Verification items for the finished model (mm, model axes). A direction names the side the tool comes from. Round coordinates to 2 decimals unless told otherwise and drop trailing zeros. Write each loop counter-clockwise with the first axis right and the second up, starting at its lowest first coordinate (ties: lowest second). Pieces come first, ordered by that corner, then holes. Notation, with made-up numbers: (43.5, 74) -> (49.5, 74) arc R23 ccw to (49.5, 96) -> close; hole circle Ø4 at (50, -27). An arc over 180 degrees is marked (long way). Use CSV: the item, a comma, the result in double quotes.
Autodesk Inventor part; units mm, degrees
ref_plane "YZ Plane" through (0, 0, 0) normal (1, 0, 0) x (0, 1, 0)
ref_plane "XZ Plane" through (0, 0, 0) normal (0, 1, 0) x (-1, 0, 0)
ref_plane "XY Plane" through (0, 0, 0) normal (0, 0, 1) x (1, 0, 0)
sketch "Sketch1" plane through (0, 0, 0) normal (0, 1, 0) x (-1, 0, 0)
  line L0 (-20, 10) -> (20, 10)
  line L1 (20, 10) -> (20, -10)
  line L2 (20, -10) -> (-20, -10)
  line L3 (-20, -10) -> (-20, 10)
  line L4 (-20, 10) -> (20, -10) construction
  line L5 (20, 10) -> (-20, -10) construction
  point P0 (0, 0)
  dimension "d0" = 40
  dimension "d1" = 20
extrude "Extrusion1" add sketch "Sketch1" along normal blind 15
sketch "Sketch2" plane through (0, 15, 0) normal (0, 1, 0) x (1, 0, 0)
  line L0 (20, 10) -> (-20, 10) construction
  line L1 (-20, -10) -> (20, -10) construction
  line L2 (20, -10) -> (20, 10) construction
  line L3 (20, 10) -> (-20, 10) construction
  line L4 (-20, 10) -> (-20, -10) construction
  line L5 (-20, -10) -> (20, 10) construction
  line L6 (20, -10) -> (-20, 10) construction
  line L7 (-10, -5) -> (10, -5) construction
  line L8 (10, -5) -> (10, 5) construction
  line L9 (10, 5) -> (-10, 5) construction
  line L10 (-10, 5) -> (-10, -5) construction
  line L11 (-10, -5) -> (10, 5) construction
  line L12 (10, -5) -> (-10, 5) construction
  point P0 (0, 0)
  dimension "d4" = 20
hole "Hole1" at (-10, 15, -5) at (-10, 15, 5) at (10, 15, 5) at (10, 15, -5) direction (0, -1, 0) diameter 4 end through all counterbore diameter 6 counterbore depth 1
fillet "Fillet1" radius 2 1 edges at (0, 0, 10)
sketch "Sketch3" plane through (20, 0, -10) normal (1, 0, 0) x (0, 0, -1)
  line L0 (0, 0) -> (0, 15)
  line L1 (0, 15) -> (5, 15)
  line L2 (5, 15) -> (5, -15)
  line L3 (5, -15) -> (0, -15)
  line L4 (0, -15) -> (0, 15)
  point P0 (-10, 0)
  dimension "d13" = 5
  dimension "d14" = 30
extrude "Extrusion2" add sketch "Sketch3" against normal up to surface (40 mm away)
sketch "Sketch4" plane through (20, -15, -15) normal (0, 0, -1) x (-1, 0, 0)
  line L0 (0, 17) -> (0, 30)
  line L1 (0, 0) -> (40, 0)
  line L2 (0, 30) -> (40, 30)
  line L3 (40, 30) -> (40, 0)
  line L4 (40, 0) -> (0, 0)
  line L5 (0, 0) -> (0, 30)
  point P0 (20, 15)
extrude "Extrusion3" add sketch "Sketch4" along normal blind 10
sketch "Sketch5" plane through (20, -15, -25) normal (0, 0, -1) x (-1, 0, 0)
  point P0 (20, 15)
  point P1 (20, 15)
hole "Hole2" at (0, 0, -25) direction (0, 0, 1) diameter 7.5 depth 10
sketch "Sketch6" plane through (20, -15, -25) normal (0, 0, -1) x (-1, 0, 0)
  point P0 (20, 15)
  point P1 (20, 15)
hole "Hole3" at (0, 0, -25) direction (0, 0, 1) diameter 19.2 depth 6.5
sketch "Sketch7" plane through (20, -15, -25) normal (0, 0, -1) x (-1, 0, 0)
  line L0 (40, 0) -> (40, 30)
  line L1 (40, 30) -> (0, 30)
  line L2 (40, 0) -> (32, 0)
  line L3 (32, 0) -> (32, 30)
  line L4 (32, 30) -> (40, 30)
  line L5 (40, 30) -> (40, 0)
  line L6 (0, 0) -> (40, 0) construction
  line L7 (20, 0) -> (20, 30) construction
  line L8 (0, 0) -> (0, 30)
  line L9 (0, 0) -> (8, 0)
  line L10 (8, 0) -> (8, 30)
  line L11 (8, 30) -> (0, 30)
  line L12 (0, 30) -> (0, 0)
  point P0 (20, 15)
  dimension "d33" = 8
extrude "Extrusion4" add sketch "Sketch7" along normal blind 10
sketch "Sketch8" plane through (20, -15, -35) normal (0, 0, -1) x (-1, 0, 0)
  line L0 (40, 15) -> (40, 0)
  line L1 (40, 30) -> (0, 30)
  line L2 (40, 0) -> (0, 0)
  line L3 (0, 0) -> (0, 30)
  line L4 (0, 30) -> (40, 30)
  line L5 (40, 30) -> (40, 0)
  point P0 (20, 15)
extrude "Extrusion5" add sketch "Sketch8" along normal blind 10
sketch "Sketch9" plane through (20, -15, -45) normal (0, 0, -1) x (-1, 0, 0)
  line L0 (40, 15) -> (40, 0) construction
  line L1 (0, 17) -> (0, 30) construction
  line L2 (40, 0) -> (0, 30) construction
  line L3 (40, 17) -> (40, 30) construction
  line L4 (0, 0) -> (0, 15) construction
  line L5 (40, 30) -> (0, 0) construction
  point P0 (20, 15)
  point P1 (20, 15)
hole "Hole4" at (0, 0, -45) direction (0, 0, 1) diameter 7.5 depth 10 counterbore diameter 19.2 counterbore depth 6
sketch "Sketch10" plane through (-20, 2, 10) normal (-1, 0, 0) x (0, 0, 1)
  line L0 (-55, -17) -> (-55, 13) construction
  line L1 (-55, 13) -> (-45, 13) construction
  line L2 (-45, 13) -> (-45, 8) construction
  line L3 (-45, 8) -> (-55, 8) construction
  line L4 (-55, 8) -> (-55, 13) construction
  line L5 (-55, 13) -> (-35, 13) construction
  line L6 (-35, 13) -> (-35, 8) construction
  line L7 (-35, 8) -> (-55, 8) construction
  line L8 (-55, 8) -> (-55, 13) construction
  point P0 (-10, -2)
  dimension "d45" = 10
  dimension "d46" = 5
  dimension "d47" = 20
hole "Hole5" at (-20, 10, -35) at (-20, 10, -25) direction (1, 0, 0) diameter 5 depth 6 tip angle 118 countersink diameter 6.5 countersink angle 90
mirror "Mirror1" about plane through (0, 0, 0) normal (1, 0, 0) of "Hole5"
fillet "Fillet2" radius 1 6 edges at (-20, 15, -17.5) (-20, 0.5858, 9.4142) (-20, 0, -1) (-20, 8.5, 10) (-20, -7.5, -10) (-20, 0, -45)
properties part number "Swivel Joint Driver"
Q1. Section check A-A (z = -5). Record the cut outline in (x, y).
Filled in:
outline,"(-20, 1) arc R1 ccw to (-19, 0) -> (-12, 0) -> (-12, 14) -> (-13, 14) -> (-13, 15) -> (-19, 15) arc R1 ccw to (-20, 14) -> close; (-8, 0) -> (8, 0) -> (8, 14) -> (7, 14) -> (7, 15) -> (-7, 15) -> (-7, 14) -> (-8, 14) -> close; (12, 0) -> (20, 0) -> (20, 15) -> (13, 15) -> (13, 14) -> (12, 14) -> close"
Q2. Section check B-B (x = 0). Record the cut outline in (y, z), plus the area to 3 significant figures.
Filled in:
outline,"(-15, -45) -> (-9.6, -45) -> (-9.6, -39) -> (-3.75, -39) -> (-3.75, -35) -> (-15, -35) -> close; (-15, -25) -> (-9.6, -25) -> (-9.6, -18.5) -> (-3.75, -18.5) -> (-3.75, -15) -> (3.75, -15) -> (3.75, -18.5) -> (9.6, -18.5) -> (9.6, -25) -> (15, -25) -> (15, 10) -> (2, 10) arc R2 ccw to (0, 8) -> (0, -10) -> (-15, -10) -> close; (3.75, -39) -> (9.6, -39) -> (9.6, -45) -> (15, -45) -> (15, -35) -> (3.75, -35) -> close"
area,"753 mm²"
Q3. Go/stop test with flat-tipped pins: P1, Ø9.5, axis at x = -10, z = 5, coming from the +Y side; P2, Ø4.5, axis at x = 10, z = -5, coming from the +Y side; P3, Ø4.5, axis at y = 10, z = -35, coming from the -X side; P4, Ø4, axis at y = 10, z = -35, coming from the +X side. Record where each tip stops, or that it passes through.
Filled in:
P1,"y = 15"
P2,"y = 14"
P3,"x = -13.85"
P4,"x = 13.7"
Q4. Material ranges on L1, parallel to Z at x = -16.1, y = 10; L2, parallel to Z at x = -7.5, y = -8.5; L3, parallel to X at y = 0, z = -16, recorded low to high.
Filled in:
L1,"-45 to -37.5, -32.5 to -27.5, -22.5 to 10"
L2,"-45 to -35, -25 to -10"
L3,"-20 to -3.75, 3.75 to 20"
Q5. Section check D-D (z = -20.5). Record the cut outline in (x, y), plus the area to 3 significant figures.
Filled in:
outline,"(-20, -15) -> (20, -15) -> (20, 15) -> (-19, 15) arc R1 ccw to (-20, 14) -> close; hole circle Ø19.2 at (0, 0)"
area,"910 mm²"
Q6. Section check C-C (y = -13). Record the cut outline in (x, z).
Filled in:
outline,"(-20, -44) arc R1 ccw to (-19, -45) -> (20, -45) -> (20, -10) -> (-19, -10) arc R1 ccw to (-20, -11) -> close; hole (-12, -35) -> (12, -35) -> (12, -25) -> (-12, -25) -> close"
Q7. Mould release check, pull along Y, two halves, no side actions. Record for faces 4 (the flat face through (1, 0, -1)), 5 (the flat face through (9.4, -3.1, -45)), 6 (the conical face through (-12.759, 9.736, -35.345)): released by +Y, released by -Y, zero draft, split by the parting line, or undercut.
Filled in:
face 4,"released by -Y"
face 5,"zero draft"
face 6,"undercut"
Q8. Access from +Z, -Z, +X, -X, +Y, -Y to the whole of each face (thin tool, end or side, straight path). Record for faces 1 (the flat face through (4, 0, -18.5)), 2 (the cylindrical face through (-8.095, 5.161, -41.958)), 3 (the cylindrical face through (16.59, 9.04, -32.69)).
Filled in:
face 1,"none"
face 2,"-Z"
face 3,"+X"
